from build123d import *

# Parameters (mm, degrees)
SKETCH_1_W          = 60
SKETCH_1_H          = 20
SKETCH_1_R          = 4
SKETCH_1_R_2        = 2
EXTRUDE_1_DEPTH     = 6
CUT_EXTRUDE_1_DEPTH = 3


with BuildPart() as part:
    # 草圖1 → 填料-伸長1 (new body)
    with BuildSketch(Plane.XY):
        with Locations((30, 10)):
            Rectangle(SKETCH_1_W, SKETCH_1_H)
        with Locations((7.5, 10)):
            Circle(SKETCH_1_R, mode=Mode.SUBTRACT)
        with Locations((17.5, 10)):
            Circle(SKETCH_1_R_2, mode=Mode.SUBTRACT)
        with Locations((25.5, 10)):
            Circle(SKETCH_1_R_2, mode=Mode.SUBTRACT)
        with Locations((52.5, 10)):
            Circle(SKETCH_1_R, mode=Mode.SUBTRACT)
    extrude(amount=EXTRUDE_1_DEPTH)

    # 草圖3 → 除料-伸長1 (cut)
    with BuildSketch(Plane(origin=(0, 0, 0), x_dir=(-1, 0, 0), z_dir=(0, 0, -1))):
        with BuildLine():
            Line((-25.5, 12.75), (-17.5, 12.75))
            ThreePointArc((-17.5, 12.75), (-14.75, 10), (-17.5, 7.25))
            Line((-17.5, 7.25), (-25.5, 7.25))
            ThreePointArc((-25.5, 7.25), (-28.25, 10), (-25.5, 12.75))
        make_face()
    extrude(amount=-CUT_EXTRUDE_1_DEPTH, mode=Mode.SUBTRACT)


solid = part.part
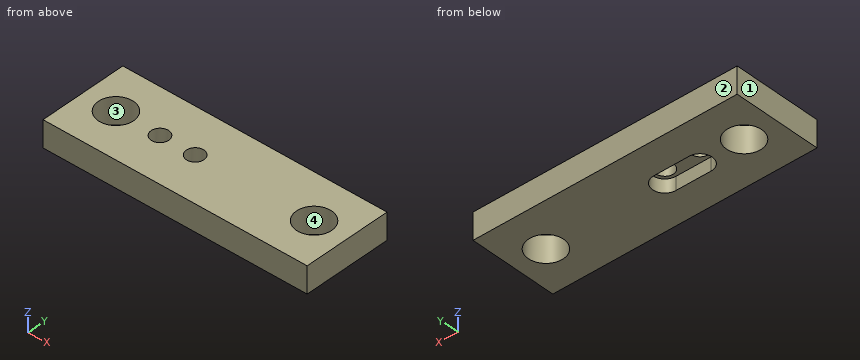
Model file for the job. Use its own axes, mm. Face numbers are marked on the shaded views. Coordinates: 2 decimals unless noted, no trailing zeros. Order: outer loops, then holes, each group sorted by start corner. A loop starts at its lowest first (then second) coordinate and runs counter-clockwise, first axis right, second up. Notation, with made-up numbers: (12.25, -9.5) -> (34.25, -9.5) arc R15 cw to (34.25, -1.5) -> close; hole circle Ø1 at (37, 85.5). An arc over 180 degrees is marked (long way). Return JSON: item names as keys, results as strings. Group by question number.
Item 1: Wall check: line 1 along Y through (x, z) = (17.5, 4.6); line 2 along Y through (x, z) = (7.5, 1.4); line 3 along X through (y, z) = (7.5, 5.7). Give the ranges that are in metal, low to high. Write a range as [from, to].
Item 2: Saw through at A-A on y = 10. Write the cut outline in (x, z), then the cut area to 4 significant figures.
Item 3: Pull direction Y, two halves, no side cores. Call the marked faces 1, 2, 3 and 4: pulls with the +Y half, pulls with the -Y half, needs draft (parallel to the pull), parting line crosses it, or undercut.
Item 4: Saw through at D-D on x = 54. Write the cut outline in (y, z), then the cut area to 3 significant figures.
Item 5: Saw through at C-C on z = 0.95. Write the cut outline in (x, y).
Item 6: Saw through at B-B on z = 4.5. Write the cut outline in (x, y), then the cut area to 3 significant figures.
Item 7: Flat gauge pin, fed straight in: P1, Ø4.5, axis at x = 21, y = 10, coming from the -Z side. Where does the tip first touch, or does it go through?
Values found:
{
 "1": {"line 1": "y = [0, 8], [12, 20]", "line 2": "y = [0, 6], [14, 20]", "line 3": "x = [0, 4.38], [10.62, 49.38], [55.62, 60]"},
 "2": {"outline": "(0, 0) -> (3.5, 0) -> (3.5, 6) -> (0, 6) -> close; (11.5, 0) -> (14.75, 0) -> (14.75, 3) -> (15.5, 3) -> (15.5, 6) -> (11.5, 6) -> close; (19.5, 3) -> (23.5, 3) -> (23.5, 6) -> (19.5, 6) -> close; (27.5, 3) -> (28.25, 3) -> (28.25, 0) -> (48.5, 0) -> (48.5, 6) -> (27.5, 6) -> close; (56.5, 0) -> (60, 0) -> (60, 6) -> (56.5, 6) -> close", "area": "199.5 mm2"},
 "3": {"face 1": "needs draft", "face 2": "pulls with the +Y half", "face 3": "undercut", "face 4": "undercut"},
 "4": {"outline": "(0, 0) -> (6.29, 0) -> (6.29, 6) -> (0, 6) -> close; (13.71, 0) -> (20, 0) -> (20, 6) -> (13.71, 6) -> close", "area": "75.5 mm2"},
 "5": {"outline": "(0, 0) -> (60, 0) -> (60, 20) -> (0, 20) -> close; hole circle Ø8 at (7.5, 10); hole (17.5, 7.25) -> (25.5, 7.25) arc R2.75 ccw to (25.5, 12.75) -> (17.5, 12.75) arc R2.75 ccw to start; hole circle Ø8 at (52.5, 10)"},
 "6": {"outline": "(0, 0) -> (60, 0) -> (60, 20) -> (0, 20) -> close; hole circle Ø8 at (7.5, 10); hole circle Ø4 at (17.5, 10); hole circle Ø4 at (25.5, 10); hole circle Ø8 at (52.5, 10)", "area": "1,070 mm2"},
 "7": {"P1": "stops at z = 3"}
}
